For this review, take the finished solid that the model builds, in its own axes (mm). A direction names the side the tool comes from. Give positions to 0.01 mm unless a question says otherwise; leave off trailing zeros. Order: outer loops, then holes, each group sorted by start corner. A loop starts at its lowest first (then second) coordinate and runs counter-clockwise, first axis right, second up. Notation, with made-up numbers: M 14.5,78 L 55.5,78 A14 ccw 55.5,83 Z; hole C 82.25,80 d8. An arc over 180 degrees is marked long. Answer as CSV lines item,"result". Start each with the question number.
1. Machinability: for faces 1 (the flat face through (0, 0, 2.54)), 2 (the cylindrical face through (-6.486, -0.681, 1.288)), which of the approach directions +Z, -Z, +X, -X, +Y, -Y give a long, thin tool a straight path to every point of the face, cutting with its end or side? Answer none if there is none.
2. We need section C-C, the plane x = -4. Give the boundary of the cut face in (y, z), and give its area (3 significant figures).
3. For line 1 along Y through (x, z) = (0, 0.6) (3 decimals); line 2 along Y through (x, z) = (0, 46); line 3 along Z through (x, y) = (1, -11), list the stretches that pass through material, from the lowest coordinate up.
4. We need section A-A, the plane y = 0. State how many separate pieces and enclosed holes the cut face has, and give its area (3 significant figures).
5. We need section B-B, the plane z = 142.5. Give the boundary of the cut face in (x, y) (1 decimal), and give its area (3 significant figures).
6. Mouldability with a two-part tool opening along Y and no side actions: class faces 3 (the cylindrical face through (6.35, 0.08, 1.29)), 4 (the cylindrical face through (-3.441, -15.497, 1.252)), 5 (the flat face through (-5, 12, 2.54)) as pulls with the +Y half, pulls with the -Y half, needs draft (parallel to the pull), parting line crosses it, or undercut.
7. Clearance check with flat-ended pins moving along their axes: P1, Ø5, axis at x = 8.5, z = 170.5, coming from the +Y side; P2, Ø4, axis at x = 4.5, y = 5, coming from the +Z side; P3, Ø1, axis at y = 10.5, z = 52, coming from the -X side. State where each tip first meets the part, or that it passes through.
from build123d import *

# Parameters (mm, degrees)
SKETCH1_R           = 15.875
BOSS_EXTRUDE1_DEPTH = 2.54
SKETCH2_R           = 12.7
SKETCH2_R_2         = 11.1125
BOSS_EXTRUDE2_DEPTH = 203.2
SKETCH3_R           = 1.778
CUT_EXTRUDE1_DEPTH  = 2.54
SKETCH4_R           = 0.9271
CUT_EXTRUDE2_DEPTH  = 2.54


with BuildPart() as part:
    # Sketch1 → Boss-Extrude1 (new body)
    with BuildSketch(Plane.XY):
        Circle(SKETCH1_R)
    extrude(amount=BOSS_EXTRUDE1_DEPTH)

    # Sketch2 → Boss-Extrude2 (add)
    with BuildSketch(Plane.XY.offset(2.54)):
        Circle(SKETCH2_R)
        Circle(SKETCH2_R_2, mode=Mode.SUBTRACT)
    extrude(amount=BOSS_EXTRUDE2_DEPTH)

    # Sketch3 → Cut-Extrude1 (cut)
    with BuildSketch(Plane.XY.offset(2.54)):
        with Locations((-8.128, 0)):
            Circle(SKETCH3_R)
        with Locations((8.128, 0)):
            Circle(SKETCH3_R)
    extrude(amount=-CUT_EXTRUDE1_DEPTH, mode=Mode.SUBTRACT)

    # Sketch4 → Cut-Extrude2 (cut)
    with BuildSketch(Plane.XY.offset(2.54)):
        with Locations((0, 14.2875)):
            Circle(SKETCH4_R)
        with Locations((0, -14.2875)):
            Circle(SKETCH4_R)
    extrude(amount=-CUT_EXTRUDE2_DEPTH, mode=Mode.SUBTRACT)


solid = part.part
Result set:
1,face 1,"+Z"
1,face 2,"+Z, -Z"
2,outline,"M -15.36,0 L 15.36,0 L 15.36,2.54 L 12.05,2.54 L 12.05,205.74 L 10.37,205.74 L 10.37,2.54 L -10.37,2.54 L -10.37,205.74 L -12.05,205.74 L -12.05,2.54 L -15.36,2.54 Z"
2,area,"763 mm2"
3,line 1,"-15.875 to -15.215, -13.36 to 13.36, 15.215 to 15.875"
3,line 2,"-12.7 to -11.11, 11.11 to 12.7"
3,line 3,"0 to 2.54"
4,separate pieces,"3"
4,enclosed holes,"0"
4,area,"708 mm2"
5,outline,"C 0,0 d25.4; hole C 0,0 d22.2"
5,area,"119 mm2"
6,face 3,"undercut"
6,face 4,"parting line crosses it"
6,face 5,"needs draft"
7,P1,"y = 11.19"
7,P2,"z = 2.54"
7,P3,"x = -7.83"
